Design review of the part built by this model. Coordinates are the model's own, in mm. A direction names the side the tool comes from. Coordinates: 2 decimals unless noted, no trailing zeros. Order: outer loops, then holes, each group sorted by start corner. A loop starts at its lowest first (then second) coordinate and runs counter-clockwise, first axis right, second up. Notation, with made-up numbers: (68.5, 76.25) -> (119.5, 76.25) arc R14 cw to (119.5, 98.25) -> close; hole circle Ø1 at (35, 35.5). An arc over 180 degrees is marked (long way). Use a Markdown table: item, result. Add a question column.
Q1. Add section C-C (y = 28.5). State the section outline as (x, z) points.
Q2. Add section A-A (z = 2.25). State the section outline as (x, y) points.
Q3. The part is to be moulded in two halves that separate along X. For faces 3 (the face through (-54.72, -96.01, 1.48)), 4 (the face through (-1, 21, 0)), say which applies: pulls with the +X half, pulls with the -X half, needs draft (parallel to the pull), parting line crosses it, or undercut.
Q4. Add section D-D (x = 55). State the section outline as (y, z) points.
Q5. Add section B-B (x = 32). State the section outline as (y, z) points, then the cut area to 3 significant figures.
Q6. Wall thickness on probe 1 along X at (y, z) = (-1, 2.55); probe 2 along Y at (x, z) = (-34, 2.7); probe 3 along Y at (x, z) = (-56, 0.15): over which ranges is each line inside the solid? List them lowest first.
Q7. Insertion check: pin 1 (1.5 mm diameter, centred on y = 40.5, z = 1, fed in from -X); pin 2 (0.9 mm diameter, centred on x = -13, z = 2, fed in from -Y); pin 3 (1.5 mm diameter, centred on y = 26, z = 1.5, fed in from +X). Each pin has a flat end and moves straight along its axis. Give the tip position at first contact, or say it passes through.
Q8. Machinability: for faces 1 (the face through (-1, 21, 3)), 2 (the face through (54.49, -95.78, 1.48)), which of the approach directions +Z, -Z, +X, -X, +Y, -Y give a long, thin tool a straight path to every point of the face, cutting with its end or side? Answer none if there is none.
Autodesk Inventor part; units mm, degrees
ref_plane "YZ Plane" through (0, 0, 0) normal (1, 0, 0) x (0, 1, 0)
ref_plane "XZ Plane" through (0, 0, 0) normal (0, 1, 0) x (-1, 0, 0)
ref_plane "XY Plane" through (0, 0, 0) normal (0, 0, 1) x (1, 0, 0)
sketch "Sketch1" plane through (0, 0, 0) normal (0, 0, 1) x (1, 0, 0)
  line L0 (-84, -131.5) -> (84, -131.5)
  line L1 (84, -131.5) -> (84, 168.5)
  line L2 (84, 168.5) -> (-84, 168.5)
  line L3 (-84, 168.5) -> (-84, -131.5)
  line L4 (-84, 1.5) -> (-84, -1.5)
  line L5 (84, -1.5) -> (84, 1.5)
  line L6 (61, -1.5) -> (84, -1.5)
  line L7 (26, -1.5) -> (61, -1.5)
  line L8 (61, 1.5) -> (61, -1.5)
  line L9 (26, 1.5) -> (61, 1.5)
  line L10 (26, 1.5) -> (26, -1.5)
  point P0 (0, 0)
  dimension "d0" = 300
  dimension "d1" = 170
extrude "Extrusion1" add sketch "Sketch1" along normal blind 3
sketch "Sketch2" plane through (0, 0, 0) normal (0, 0, -1) x (-1, 0, 0)
  line L0 (84, 1.5) -> (84, -1.5)
  line L1 (84, -1.5) -> (61, -1.5)
  line L2 (61, 1.5) -> (61, -1.5)
  line L3 (26, 1.5) -> (61, 1.5)
  line L4 (26, -1.5) -> (26, 1.5)
  line L5 (26, -1.5) -> (-26, -1.5)
  line L6 (-26, 1.5) -> (-26, -1.5)
  line L7 (-61, 1.5) -> (-26, 1.5)
  line L8 (-61, -1.5) -> (-61, 1.5)
  line L9 (-61, -1.5) -> (-84, -1.5)
  line L10 (-84, -1.5) -> (-84, 1.5)
  line L11 (-84, 1.5) -> (-61, 1.5)
  line L12 (61, 1.5) -> (84, 1.5)
  line L13 (61, -1.5) -> (26, -1.5)
  line L14 (-26, 1.5) -> (26, 1.5)
  line L15 (-26, -1.5) -> (-61, -1.5)
  point P0 (0, 0)
extrude "Extrusion2" cut sketch "Sketch2" against normal blind 10 contours L2 L13 L4 L3
sketch "Sketch3" plane through (0, 0, 3) normal (0, 0, 1) x (1, 0, 0)
  line L0 (84, -131.5) -> (84, 168.5)
  line L1 (84, -131.5) -> (87, -131.5)
  line L2 (87, -131.5) -> (87, -31.5)
  line L3 (87, -31.5) -> (84, -31.5)
  line L4 (84, -31.5) -> (84, -131.5)
  line L5 (-61, -1.5) -> (-26, -1.5)
  line L6 (-26, -1.5) -> (-26, 1.5)
  line L7 (-26, 1.5) -> (-61, 1.5)
  line L8 (-61, 1.5) -> (-61, -1.5)
  line L9 (26, 1.5) -> (26, -1.5)
  line L10 (26, -1.5) -> (61, -1.5)
  line L11 (61, -1.5) -> (61, 1.5)
  line L12 (61, 1.5) -> (26, 1.5)
  line L13 (-84, 168.5) -> (84, 168.5)
  line L14 (84, 168.5) -> (84, -131.5)
  line L15 (84, -131.5) -> (-84, -131.5)
  line L16 (-84, -131.5) -> (-84, 168.5)
  line L17 (87, 168.5) -> (84, 168.5)
  line L18 (84, 68.5) -> (87, 68.5)
  line L19 (87, 68.5) -> (87, 168.5)
  line L20 (84, 168.5) -> (84, 68.5)
  line L21 (-84, -31.5) -> (-87, -31.5)
  line L22 (-87, -131.5) -> (-84, -131.5)
  line L23 (-84, -131.5) -> (-84, -31.5)
  line L24 (-87, -31.5) -> (-87, -131.5)
  line L25 (-84, 168.5) -> (-87, 168.5)
  line L26 (-87, 68.5) -> (-84, 68.5)
  line L27 (-84, 68.5) -> (-84, 168.5)
  line L28 (-87, 168.5) -> (-87, 68.5)
  point P0 (0, 0)
  dimension "d6" = 100
  dimension "d7" = 3
  dimension "d10" = 200
  dimension "d13" = 171
extrude "Extrusion3" add sketch "Sketch3" against normal up to surface (3 mm away) contours L0 L3 L2 L1 | L22 L24 L21 L16 | L0 L17 L19 L18 | L26 L28 L25 L16
sketch "Sketch4" plane through (0, 0, 3) normal (0, 0, 1) x (1, 0, 0)
  line L0 (-59, -131.5) -> (59, -131.5)
  line L1 (59, -131.5) -> (59, -91.5)
  line L2 (59, -91.5) -> (-59, -91.5)
  line L3 (-59, -91.5) -> (-59, -131.5)
  line L4 (-87, -131.5) -> (87, -131.5)
  line L5 (87, -131.5) -> (87, -31.5)
  line L6 (-87, -31.5) -> (-87, -131.5)
  point P0 (0, 0)
  dimension "d18" = 28
  dimension "d19" = 28
  dimension "d20" = 40
extrude "Extrusion4" cut sketch "Sketch4" against normal blind 10
fillet "Fillet1" radius 15 2 edges at (59, -91.5, 1.5) (-59, -91.5, 1.5)
properties part number "Pared_Lateral"
Established:
| question | item | result |
|---|---|---|
| 1 | outline | (-84, 0) -> (84, 0) -> (84, 3) -> (-84, 3) -> close |
| 2 | outline | (-87, -131.5) -> (-59, -131.5) -> (-59, -106.5) arc R15 cw to (-44, -91.5) -> (44, -91.5) arc R15 cw to (59, -106.5) -> (59, -131.5) -> (87, -131.5) -> (87, -31.5) -> (84, -31.5) -> (84, 68.5) -> (87, 68.5) -> (87, 168.5) -> (-87, 168.5) -> (-87, 68.5) -> (-84, 68.5) -> (-84, -31.5) -> (-87, -31.5) -> close; hole (-61, -1.5) -> (-26, -1.5) -> (-26, 1.5) -> (-61, 1.5) -> close; hole (26, -1.5) -> (61, -1.5) -> (61, 1.5) -> (26, 1.5) -> close |
| 3 | face 3 | undercut |
| 3 | face 4 | needs draft |
| 4 | outline | (-96.3, 0) -> (-1.5, 0) -> (-1.5, 3) -> (-96.3, 3) -> close; (1.5, 0) -> (168.5, 0) -> (168.5, 3) -> (1.5, 3) -> close |
| 5 | outline | (-91.5, 0) -> (-1.5, 0) -> (-1.5, 3) -> (-91.5, 3) -> close; (1.5, 0) -> (168.5, 0) -> (168.5, 3) -> (1.5, 3) -> close |
| 5 | area | 771 mm^2 |
| 6 | probe 1 | -84 to -61, -26 to 26, 61 to 84 |
| 6 | probe 2 | -91.5 to -1.5, 1.5 to 168.5 |
| 6 | probe 3 | -97.5 to -1.5, 1.5 to 168.5 |
| 7 | pin 1 | x = -84 |
| 7 | pin 2 | y = -91.5 |
| 7 | pin 3 | x = 84 |
| 8 | face 1 | +Z, +X, -X, +Y, -Y |
| 8 | face 2 | +Z, -Z, -Y |
